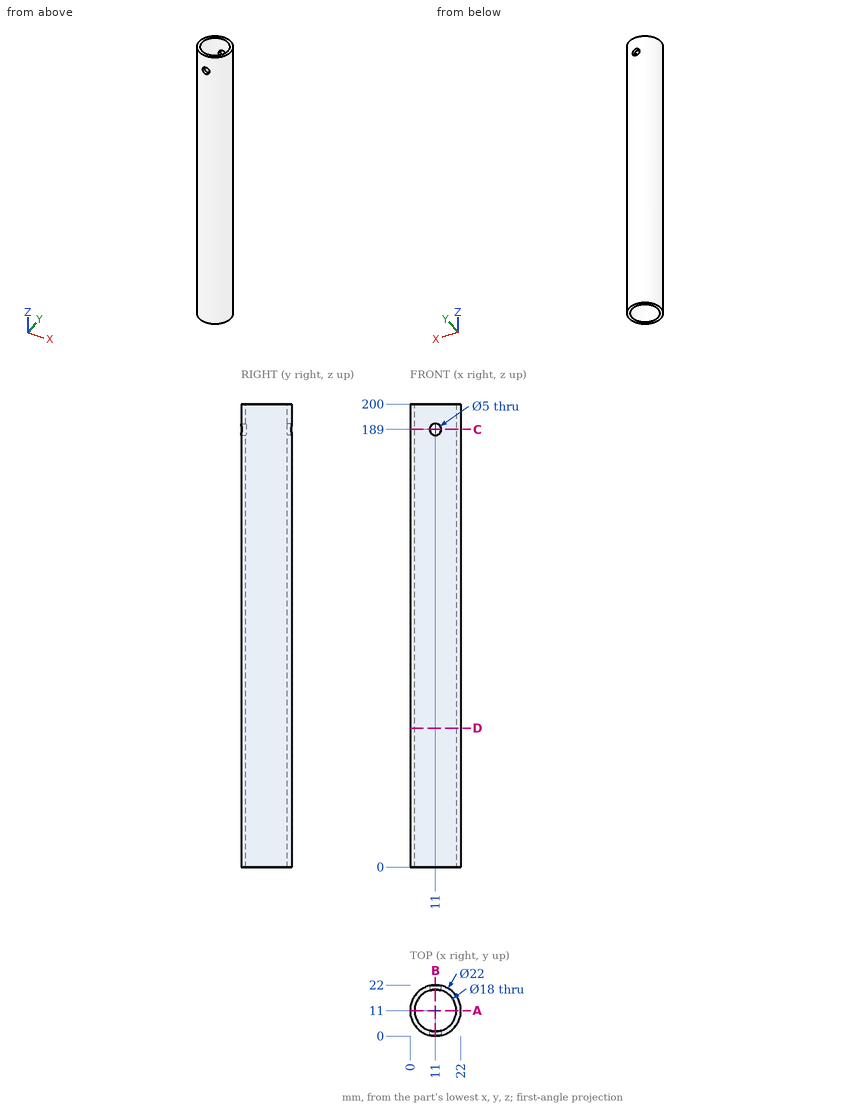
Input: dimensioned drawing with shaded views. Units: mm. Origin: part minimum x, y, z. Give positions to 0.01 mm unless a question says otherwise; leave off trailing zeros. Order: outer loops, then holes, each group sorted by start corner. A loop starts at its lowest first (then second) coordinate and runs counter-clockwise, first axis right, second up. Notation, with made-up numbers: (63, -24) -> (112, -24) arc R15 cw to (112, -13) -> close; hole circle Ø9 at (-21, 62.25). An arc over 180 degrees is marked (long way). Use one line per item in the form item = value.
1) Line query: probe 1 along Y at (x, z) = (11, 67); probe 2 along Z at (x, y) = (11, 1.75); probe 3 along Y at (x, z) = (5.25, 55.5). Output: solid intervals per line, ascending.
Response values:
probe_1 = 0 to 2, 20 to 22
probe_2 = 0 to 186.5, 191.5 to 200
probe_3 = 1.62 to 4.08, 17.92 to 20.38
2) Section B-B, the plane x = 11. Return loops of the section in (y, z).
Response values:
outline = (0, 0) -> (2, 0) -> (2, 186.5) -> (0, 186.5) -> close; (0, 191.5) -> (2, 191.5) -> (2, 200) -> (0, 200) -> close; (20, 0) -> (22, 0) -> (22, 186.5) -> (20, 186.5) -> close; (20, 191.5) -> (22, 191.5) -> (22, 200) -> (20, 200) -> close
3) Section D-D, the plane z = 60. Return loops of the section in (x, y).
Response values:
outline = circle Ø22 at (11, 11); hole circle Ø18 at (11, 11)
4) First-contact query: pin 1 Ø2 at (x, z) = (9.5, 50) entering from +Y; pin 2 Ø8 at (y, z) = (2.5, 127.5) entering from -X; pin 3 Ø4 at (x, z) = (14.5, 64.5) entering from +Y. Flat tips, straight axial feed; report the tip coordinate or a pass-through.
Response values:
pin_1 = 21.99
pin_2 = 0.96
pin_3 = 21.9
5) Section C-C, the plane z = 189. Return loops of the section in (x, y), and give its area (3 significant figures).
Response values:
outline = (8.5, 0.29) -> (8.5, 2.35) arc R9 cw to (8.5, 19.65) -> (8.5, 21.71) arc R11 ccw to start; (13.5, 0.29) arc R11 ccw to (13.5, 21.71) -> (13.5, 19.65) arc R9 cw to (13.5, 2.35) -> close
area = 105 mm^2
6) Section A-A, the plane y = 11. Return loops of the section in (x, z).
Response values:
outline = (0, 0) -> (2, 0) -> (2, 200) -> (0, 200) -> close; (20, 0) -> (22, 0) -> (22, 200) -> (20, 200) -> close
